Source: CAD feature listing. Evaluate the final solid. Frame: model axes, mm. Round coordinates to 2 decimals unless told otherwise and drop trailing zeros. Write each loop counter-clockwise with the first axis right and the second up, starting at its lowest first coordinate (ties: lowest second). Pieces come first, ordered by that corner, then holes. Notation, with made-up numbers: M 53.5,67.5 L 59.5,67.5 A23 ccw 59.5,88.5 Z; hole C 86,35 d11. An arc over 180 degrees is marked long. Answer in a Markdown table with one row per item.
Solid Edge part; units mm, degrees
sketch "Sketch1" plane through (0, 0, 0) normal (0, 0, 1) x (1, 0, 0)
  line L0 (-70.3853, 35.6849) -> (-103.7021, 94.9149)
  arc A0 (-103.2087, 98.507) -> (-103.7021, 94.9149) centre (-101.0874, 96.3857) ccw
  line L1 (-103.2087, 98.507) -> (-98.507, 103.2087)
  arc A1 (-98.507, 103.2087) -> (-94.9149, 103.7021) centre (-96.3857, 101.0874) cw
  line L2 (-94.9149, 103.7021) -> (-35.6849, 70.3853)
  arc A2 (-35.6849, 70.3853) -> (-34.2141, 70) centre (-34.2141, 73) ccw
  line L3 (-34.2141, 70) -> (34.2141, 70)
  arc A3 (34.2141, 70) -> (35.6849, 70.3853) centre (34.2141, 73) ccw
  line L4 (35.6849, 70.3853) -> (94.9149, 103.7021)
  arc A4 (94.9149, 103.7021) -> (98.507, 103.2087) centre (96.3857, 101.0874) cw
  line L5 (98.507, 103.2087) -> (103.2087, 98.507)
  arc A5 (103.2087, 98.507) -> (103.7021, 94.9149) centre (101.0874, 96.3857) cw
  line L6 (103.7021, 94.9149) -> (70.3853, 35.6849)
  arc A6 (70.3853, 35.6849) -> (70, 34.2141) centre (73, 34.2141) ccw
  line L7 (70, 34.2141) -> (70, -34.2141)
  arc A7 (70, -34.2141) -> (70.3853, -35.6849) centre (73, -34.2141) ccw
  line L8 (70.3853, -35.6849) -> (103.7021, -94.9149)
  arc A8 (103.7021, -94.9149) -> (103.2087, -98.507) centre (101.0874, -96.3857) cw
  line L9 (103.2087, -98.507) -> (98.507, -103.2087)
  arc A9 (98.507, -103.2087) -> (94.9149, -103.7021) centre (96.3857, -101.0874) cw
  line L10 (94.9149, -103.7021) -> (35.6849, -70.3853)
  arc A10 (34.2141, -70) -> (35.6849, -70.3853) centre (34.2141, -73) cw
  line L11 (34.2141, -70) -> (-34.2141, -70)
  arc A11 (-34.2141, -70) -> (-35.6849, -70.3853) centre (-34.2141, -73) ccw
  line L12 (-35.6849, -70.3853) -> (-94.9149, -103.7021)
  arc A12 (-94.9149, -103.7021) -> (-98.507, -103.2087) centre (-96.3857, -101.0874) cw
  line L13 (-98.507, -103.2087) -> (-103.2087, -98.507)
  arc A13 (-103.2087, -98.507) -> (-103.7021, -94.9149) centre (-101.0874, -96.3857) cw
  line L14 (-103.7021, -94.9149) -> (-70.3853, -35.6849)
  arc A14 (-70.3853, -35.6849) -> (-70, -34.2141) centre (-73, -34.2141) ccw
  line L15 (-70, -34.2141) -> (-70, 34.2141)
  arc A15 (-70, 34.2141) -> (-70.3853, 35.6849) centre (-73, 34.2141) ccw
extrude "Protrusion1" add sketch "Sketch1" against normal blind 6
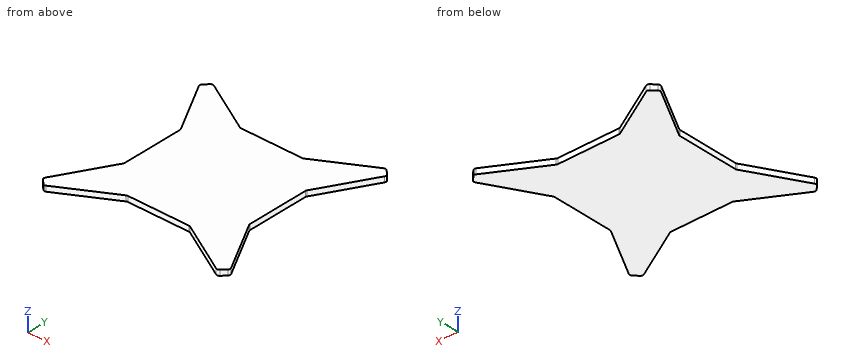
Q1. Contact query for flat-ended pins moving along their axis: pin 1 Ø2 at (y, z) = (-77.5, -4) entering from +X; pin 2 Ø3 at (y, z) = (16.5, -5) entering from +X; pin 3 Ø3 at (x, z) = (-13, -2) entering from -Y. Output: stop coordinate, or through.
Solutions:
| item | result |
|---|---|
| pin 1 | stops at x = 94.47 |
| pin 2 | stops at x = 70 |
| pin 3 | stops at y = -70 |
Q2. Section A-A (x = -78.5). Return loops of the section in (y, z).
Solutions:
| item | result |
|---|---|
| outline | M -94.47,-6 L -50.11,-6 L -50.11,0 L -94.47,0 Z; M 50.11,-6 L 94.47,-6 L 94.47,0 L 50.11,0 Z |
Q3. Section C-C (y = -85). Return loops of the section in (x, z) (3 decimals).
Solutions:
| item | result |
|---|---|
| outline | M -98.125,-6 L -61.667,-6 L -61.667,0 L -98.125,0 Z; M 61.667,-6 L 98.125,-6 L 98.125,0 L 61.667,0 Z |
Q4. Material intervals for probe 1 along Y at (x, z) = (-18.5, -0.75); probe 2 along Y at (x, z) = (83, -2.65); probe 3 along Y at (x, z) = (73, -1.9) (3 decimals), sorted ascending.
Solutions:
| item | result |
|---|---|
| probe 1 | y = -70 to 70 |
| probe 2 | y = -97 to -58.11, 58.11 to 97 |
| probe 3 | y = -91.375 to -40.333, 40.333 to 91.375 |
Q5. Section D-D (x = 7). Return loops of the section in (y, z).
Solutions:
| item | result |
|---|---|
| outline | M -70,-6 L 70,-6 L 70,0 L -70,0 Z |
